The figure shows three views and two pictorial views of one solid part (mm, origin at its lowest corner). Answer the questions. A direction names the side the tool comes from. Give positions to 0.01 mm unless a question says otherwise; leave off trailing zeros. Loops run counter-clockwise (first coordinate to the right, second up) from the corner with the lowest first, then second, coordinate; pieces in that order, holes last. Notation, with made-up numbers: (13.5, 23.25) - (68.5, 23.25) arc R19 cw to (68.5, 56.25) - close; hole circle Ø5 at (64.25, 49). An arc over 180 degrees is marked (long way). Use a Markdown table: item, result. Add a question column.
Item 1: Which of the six approach directions +Z, -Z, +X, -X, +Y, -Y give full straight-line access (tool end or side, diameter ignored) to the marked faces 4 and 5?
Item 2: This flat-tipped pin is pushed along its axis until it touches: P1, Ø4, axis at x = 34, y = 12, coming from the +Z side. Where does it stop, or does it pass through?
Item 3: Consider probe 1 along Y at (x, z) = (120.5, 15); probe 2 along X at (y, z) = (22, 8.5); probe 3 along Z at (x, y) = (75, 63.5). Determine where each line is inside the solid, lowest interval first. Write a range as [from, to].
Item 4: A cutting plane is placed at D-D (y = 72.5). Determine the outline of the cut face in (x, z).
Item 5: For a pull along X with two mould halves and no side action, classify the marked faces 1, 2 and 3 as +X half, -X half, draft (parallel to the pull), parting line (faces both ways), or undercut.
Item 6: A cutting plane is placed at A-A (z = 43.5). Determine the outline of the cut face in (x, y).
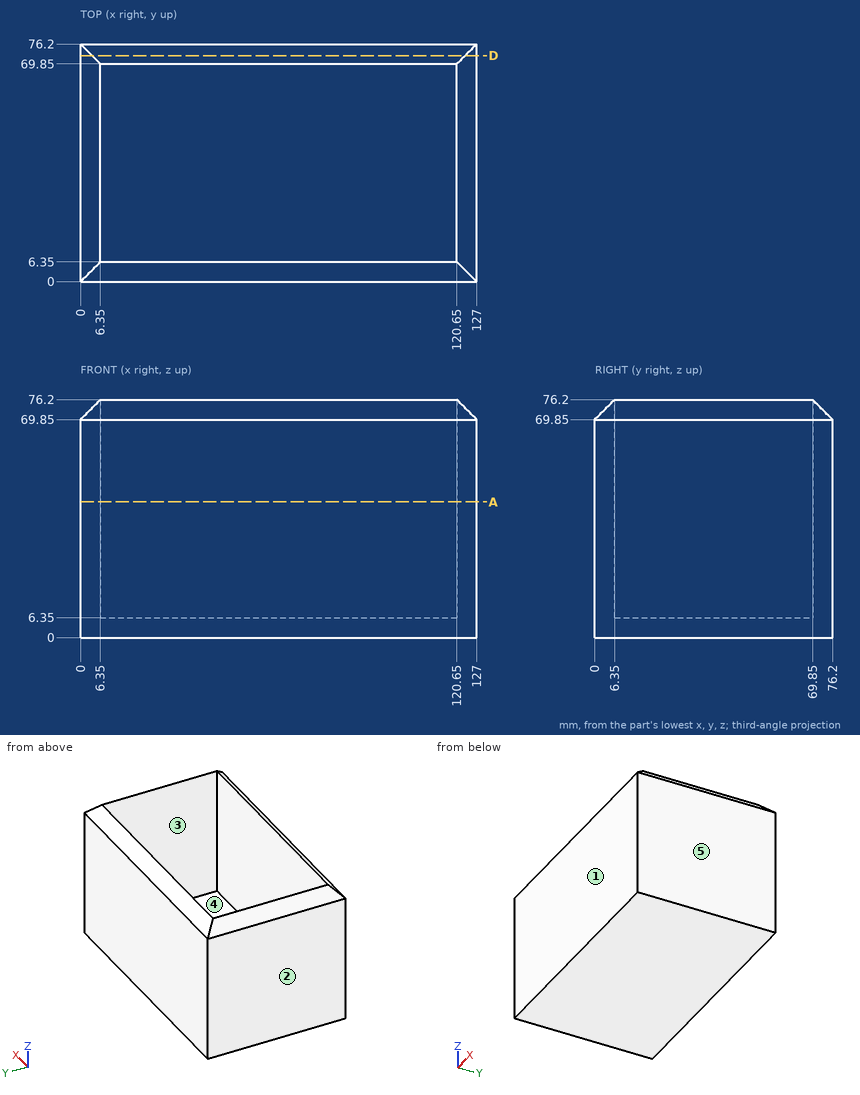
Geometry says:
| question | item | result |
|---|---|---|
| 1 | face 4 | +Z |
| 1 | face 5 | +Z, -Z, +X, +Y, -Y |
| 2 | P1 | z = 6.35 |
| 3 | probe 1 | [0, 6.35], [69.85, 76.2] |
| 3 | probe 2 | [0, 6.35], [120.65, 127] |
| 3 | probe 3 | [0, 6.35] |
| 4 | outline | (0, 0) - (127, 0) - (127, 69.85) - (123.3, 73.55) - (3.7, 73.55) - (0, 69.85) - close |
| 5 | face 1 | draft |
| 5 | face 2 | -X half |
| 5 | face 3 | undercut |
| 6 | outline | (0, 0) - (127, 0) - (127, 76.2) - (0, 76.2) - close; hole (6.35, 6.35) - (120.65, 6.35) - (120.65, 69.85) - (6.35, 69.85) - close |
